Work out the finished part from the listing and answer in its coordinate system (mm). A direction names the side the tool comes from. Coordinates: 2 decimals unless noted, no trailing zeros. Order: outer loops, then holes, each group sorted by start corner. A loop starts at its lowest first (then second) coordinate and runs counter-clockwise, first axis right, second up. Notation, with made-up numbers: M 22.5,-9 L 75.5,-9 A34 ccw 75.5,29 Z; hole C -14,-18 d3. An arc over 180 degrees is marked long. Use a Markdown table: item, result.
from build123d import *

# Parameters (mm, degrees)
F0_W     = 250
F0_H     = 60
F1_DEPTH = 1000
F2_T     = -2.5
F3_R     = 2


with BuildPart() as f1:
    # F0 (on Front) → F1 (new body)
    with BuildSketch(Plane.XZ):
        with Locations((125, 30)):
            Rectangle(F0_W, F0_H)
    extrude(amount=F1_DEPTH)

    # F2
    f2_openings = [f1.faces().sort_by_distance(p)[0] for p in [
        (125, -1000, 30),
        (125, 0, 30),
    ]]
    offset(amount=F2_T, openings=f2_openings)

    # F3
    f3_edges = [f1.edges().sort_by_distance(p)[0] for p in [
        (0, -500, 60),
        (250, -500, 60),
        (250, -500, 0),
        (0, -500, 0),
    ]]
    fillet(f3_edges, radius=F3_R)


solid = f1.part
1. Section A-A on x = 160.5 is taken. Determine the outline of the cut face in (y, z).
Answers below:
| item | result |
|---|---|
| outline | M -1000,0 L 0,0 L 0,2.5 L -1000,2.5 Z; M -1000,57.5 L 0,57.5 L 0,60 L -1000,60 Z |
2. For a pull along Z with two mould halves and no side action, classify faces 1 (the face through (123, -493, 2.5)), 2 (the face through (124, 0, 1)), 3 (the face through (123, -493, 57.5)), 4 (the face through (123, -493, 60)) as +Z half, -Z half, draft (parallel to the pull), parting line (faces both ways), or undercut.
Answers below:
| item | result |
|---|---|
| face 1 | undercut |
| face 2 | draft |
| face 3 | undercut |
| face 4 | +Z half |
3. For faces 5 (the face through (0, -493, 30)), 6 (the face through (2.5, -493, 30)), determine the directions among +Z, -Z, +X, -X, +Y, -Y from which every point of the face is accessible in a straight line to the end or side of a thin tool.
Answers below:
| item | result |
|---|---|
| face 5 | +Z, -Z, -X, +Y, -Y |
| face 6 | +Y, -Y |
4. Section C-C on y = -780 is taken. Determine the outline of the cut face in (x, z).
Answers below:
| item | result |
|---|---|
| outline | M 0,2 A2 ccw 2,0 L 248,0 A2 ccw 250,2 L 250,58 A2 ccw 248,60 L 2,60 A2 ccw 0,58 Z; hole M 2.5,2.5 L 247.5,2.5 L 247.5,57.5 L 2.5,57.5 Z |
5. Section B-B on z = 35 is taken. Determine the outline of the cut face in (x, y).
Answers below:
| item | result |
|---|---|
| outline | M 0,-1000 L 2.5,-1000 L 2.5,0 L 0,0 Z; M 247.5,-1000 L 250,-1000 L 250,0 L 247.5,0 Z |
6. Find the intervals of material crossed by probe 1 along X at (y, z) = (-749.5, 46.5); probe 2 along Z at (x, y) = (92, -901), in increasing order.
Answers below:
| item | result |
|---|---|
| probe 1 | 0 to 2.5, 247.5 to 250 |
| probe 2 | 0 to 2.5, 57.5 to 60 |
